from build123d import *

# Parameters (mm, degrees)
SKETCH2_R           = 2.15
BOSS_EXTRUDE1_DEPTH = 10.507214
CUT_EXTRUDE2_REACH  = 76.575
SKETCH4_R           = 2.15
CUT_EXTRUDE3_DEPTH  = 7
BOSS_EXTRUDE2_START = -7
SKETCH5_R           = 24.3
SKETCH5_R_2         = 23.3
BOSS_EXTRUDE2_DEPTH = 7
SKETCH6_R           = 23.3
CUT_EXTRUDE4_DEPTH  = 75.575465
CUT_EXTRUDE5_DEPTH  = 75.575465


with BuildPart() as part:
    # Sketch1 → Revolve1 (revolve)
    with BuildSketch(Plane(origin=(0, 0, 0), x_dir=(0, 0, -1), z_dir=(1, 0, 0)), mode=Mode.PRIVATE) as revolve1_sk:
        with BuildLine():
            Line((-37.5, -1.048229), (-37.5, -1.955443))
            Line((-37.5, -1.955443), (-25.283016, -1.955443))
            ThreePointArc((-25.283016, -1.955443), (-24.8, -2.421893), (-25.216498, -2.94859))
            ThreePointArc((-25.216498, -2.94859), (-25.276321, -2.982605), (-25.3, -3.04722))
            Line((-25.3, -3.04722), (-25.3, -4.555443))
            Line((-25.3, -4.555443), (-8, -4.555443))
            Line((-8, -4.555443), (-8, -11.555443))
            Line((-8, -11.555443), (-39.5, -11.555443))
            Line((-39.5, -11.555443), (-39.5, -1.048229))
            Line((-39.5, -1.048229), (-37.5, -1.048229))
        make_face()
    revolve(revolve1_sk.sketch.rotate(Axis((0, -1000, 0), (0, 1, 0)), 180), axis=Axis((0, -1000, 0), (0, 1, 0)))

    # Sketch2 → Boss-Extrude1 (add)
    # profile 1 of 4: a face of its own
    with BuildSketch(Plane.XZ.offset(11.555443)):
        with BuildLine():
            Line((-5, 47.5), (-5, 39.182266))
            Line((-5, 39.182266), (5, 39.182266))
            Line((5, 39.182266), (5, 47.5))
            ThreePointArc((5, 47.5), (0, 52.5), (-5, 47.5))
        make_face()
        with Locations(Location((0, 47.5, 0), (0, 0, 270))):
            Circle(SKETCH2_R, mode=Mode.SUBTRACT)
    # profile 2 of 4: a face of its own
    with BuildSketch(Plane.XZ.offset(11.555443)):
        with BuildLine():
            Line((47.5, -5), (39.182266, -5))
            Line((39.182266, -5), (39.182266, 5))
            Line((39.182266, 5), (47.5, 5))
            ThreePointArc((47.5, 5), (52.5, 0), (47.5, -5))
        make_face()
        with Locations(Location((47.5, 0, 0), (0, 0, 270))):
            Circle(SKETCH2_R, mode=Mode.SUBTRACT)
    # profile 3 of 4: a face of its own
    with BuildSketch(Plane.XZ.offset(11.555443)):
        with BuildLine():
            Line((-5, -47.5), (-5, -39.182266))
            Line((-5, -39.182266), (5, -39.182266))
            Line((5, -39.182266), (5, -47.5))
            ThreePointArc((5, -47.5), (0, -52.5), (-5, -47.5))
        make_face()
        with Locations(Location((0, -47.5, 0), (0, 0, 270))):
            Circle(SKETCH2_R, mode=Mode.SUBTRACT)
    # profile 4 of 4: a face of its own
    with BuildSketch(Plane.XZ.offset(11.555443)):
        with BuildLine():
            Line((-47.5, 5), (-39.182266, 5))
            Line((-39.182266, 5), (-39.182266, -5))
            Line((-39.182266, -5), (-47.5, -5))
            ThreePointArc((-47.5, -5), (-52.5, 0), (-47.5, 5))
        make_face()
        with Locations(Location((-47.5, 0, 0), (0, 0, 270))):
            Circle(SKETCH2_R, mode=Mode.SUBTRACT)
    extrude(amount=-BOSS_EXTRUDE1_DEPTH)

    # Sketch3 → Cut-Extrude2 (cut, up to next)
    with BuildSketch(Plane(origin=(0, -4.555443, 0), x_dir=(1, 0, 0), z_dir=(0, 1, 0)), mode=Mode.PRIVATE) as cut_extrude2_sk1:
        with BuildLine():
            Line((21.938323, -2), (12.369317, -2))
            ThreePointArc((12.369317, -2), (11.19262, -2.382785), (10.466345, -3.384615))
            ThreePointArc((10.466345, -3.384615), (7.778175, -7.778175), (3.384615, -10.466345))
            ThreePointArc((3.384615, -10.466345), (2.382785, -11.19262), (2, -12.369317))
            Line((2, -12.369317), (2, -21.938323))
            ThreePointArc((2, -21.938323), (2.718885, -23.474143), (4.358744, -23.905885))
            ThreePointArc((4.358744, -23.905885), (17.182695, -17.182695), (23.905885, -4.358744))
            ThreePointArc((23.905885, -4.358744), (23.474143, -2.718885), (21.938323, -2))
        make_face()
    cut_extrude2_tool1 = extrude(cut_extrude2_sk1.sketch, amount=-CUT_EXTRUDE2_REACH, mode=Mode.PRIVATE) & part.part
    # Sketch3 → Cut-Extrude2 (cut, up to next)
    with BuildSketch(Plane(origin=(0, -4.555443, 0), x_dir=(1, 0, 0), z_dir=(0, 1, 0)), mode=Mode.PRIVATE) as cut_extrude2_sk2:
        with BuildLine():
            Line((-2, -21.938323), (-2, -12.369317))
            ThreePointArc((-2, -12.369317), (-2.382785, -11.19262), (-3.384615, -10.466345))
            ThreePointArc((-3.384615, -10.466345), (-7.778175, -7.778175), (-10.466345, -3.384615))
            ThreePointArc((-10.466345, -3.384615), (-11.19262, -2.382785), (-12.369317, -2))
            Line((-12.369317, -2), (-21.938323, -2))
            ThreePointArc((-21.938323, -2), (-23.474143, -2.718885), (-23.905885, -4.358744))
            ThreePointArc((-23.905885, -4.358744), (-17.182695, -17.182695), (-4.358744, -23.905885))
            ThreePointArc((-4.358744, -23.905885), (-2.718885, -23.474143), (-2, -21.938323))
        make_face()
    cut_extrude2_tool2 = extrude(cut_extrude2_sk2.sketch, amount=-CUT_EXTRUDE2_REACH, mode=Mode.PRIVATE) & part.part
    # Sketch3 → Cut-Extrude2 (cut, up to next)
    with BuildSketch(Plane(origin=(0, -4.555443, 0), x_dir=(1, 0, 0), z_dir=(0, 1, 0)), mode=Mode.PRIVATE) as cut_extrude2_sk3:
        with BuildLine():
            Line((-21.938323, 2), (-12.369317, 2))
            ThreePointArc((-12.369317, 2), (-11.19262, 2.382785), (-10.466345, 3.384615))
            ThreePointArc((-10.466345, 3.384615), (-7.778175, 7.778175), (-3.384615, 10.466345))
            ThreePointArc((-3.384615, 10.466345), (-2.382785, 11.19262), (-2, 12.369317))
            Line((-2, 12.369317), (-2, 21.938323))
            ThreePointArc((-2, 21.938323), (-2.718885, 23.474143), (-4.358744, 23.905885))
            ThreePointArc((-4.358744, 23.905885), (-17.182695, 17.182695), (-23.905885, 4.358744))
            ThreePointArc((-23.905885, 4.358744), (-23.474143, 2.718885), (-21.938323, 2))
        make_face()
    cut_extrude2_tool3 = extrude(cut_extrude2_sk3.sketch, amount=-CUT_EXTRUDE2_REACH, mode=Mode.PRIVATE) & part.part
    # Sketch3 → Cut-Extrude2 (cut, up to next)
    with BuildSketch(Plane(origin=(0, -4.555443, 0), x_dir=(1, 0, 0), z_dir=(0, 1, 0)), mode=Mode.PRIVATE) as cut_extrude2_sk4:
        with BuildLine():
            Line((2, 21.938323), (2, 12.369317))
            ThreePointArc((2, 12.369317), (2.382785, 11.19262), (3.384615, 10.466345))
            ThreePointArc((3.384615, 10.466345), (7.778175, 7.778175), (10.466345, 3.384615))
            ThreePointArc((10.466345, 3.384615), (11.19262, 2.382785), (12.369317, 2))
            Line((12.369317, 2), (21.938323, 2))
            ThreePointArc((21.938323, 2), (23.474143, 2.718885), (23.905885, 4.358744))
            ThreePointArc((23.905885, 4.358744), (17.182695, 17.182695), (4.358744, 23.905885))
            ThreePointArc((4.358744, 23.905885), (2.718885, 23.474143), (2, 21.938323))
        make_face()
    cut_extrude2_tool4 = extrude(cut_extrude2_sk4.sketch, amount=-CUT_EXTRUDE2_REACH, mode=Mode.PRIVATE) & part.part
    add(cut_extrude2_tool1.solids().sort_by_distance((12.193258, -4.555443, 12.193258))[0], mode=Mode.SUBTRACT)
    add(cut_extrude2_tool2.solids().sort_by_distance((-12.193258, -4.555443, 12.193258))[0], mode=Mode.SUBTRACT)
    add(cut_extrude2_tool3.solids().sort_by_distance((-12.193258, -4.555443, -12.193258))[0], mode=Mode.SUBTRACT)
    add(cut_extrude2_tool4.solids().sort_by_distance((12.193258, -4.555443, -12.193258))[0], mode=Mode.SUBTRACT)

    # Sketch4 → Cut-Extrude3 (cut)
    with BuildSketch(Plane(origin=(0, -11.555443, 0), x_dir=(-1, 0, 0), z_dir=(0, -1, 0))):
        with Locations(Location((30, 0, 0), (0, 0, 90))):
            Circle(SKETCH4_R)
        with Locations(Location((0, -30, 0), (0, 0, 90))):
            Circle(SKETCH4_R)
        with Locations(Location((-30, 0, 0), (0, 0, 90))):
            Circle(SKETCH4_R)
        with Locations(Location((0, 30, 0), (0, 0, 90))):
            Circle(SKETCH4_R)
    extrude(amount=-CUT_EXTRUDE3_DEPTH, mode=Mode.SUBTRACT)

    # Sketch5 → Boss-Extrude2 (add)
    with BuildSketch(Plane.XZ.offset(11.555443).offset(BOSS_EXTRUDE2_START)):
        Circle(SKETCH5_R)
        Circle(SKETCH5_R_2, mode=Mode.SUBTRACT)
    extrude(amount=BOSS_EXTRUDE2_DEPTH)

    # Sketch6 → Cut-Extrude4 (cut, through all)
    with BuildSketch(Plane(origin=(0, -4.555443, 0), x_dir=(1, 0, 0), z_dir=(0, 1, 0))):
        with Locations(Location((0, 0, 0), (0, 0, 90))):
            Circle(SKETCH6_R)
    extrude(amount=-CUT_EXTRUDE4_DEPTH, mode=Mode.SUBTRACT)

    # Sketch7 → Cut-Extrude5 (cut, through all)
    with BuildSketch(Plane(origin=(0, -4.555443, 0), x_dir=(1, 0, 0), z_dir=(0, 1, 0))):
        with BuildLine():
            Line((11.65, 20.178392), (0, 0))
            Line((0, 0), (11.65, -20.178392))
            ThreePointArc((11.65, -20.178392), (20.178392, -11.65), (23.3, 0))
            ThreePointArc((23.3, 0), (20.178392, 11.65), (11.65, 20.178392))
        make_face()
        with BuildLine():
            Line((-11.65, -20.178392), (0, 0))
            Line((0, 0), (-11.65, 20.178392))
            ThreePointArc((-11.65, 20.178392), (-23.3, 0), (-11.65, -20.178392))
        make_face()
        with BuildLine():
            ThreePointArc((23.3, 0), (20.178392, -11.65), (11.65, -20.178392))
            Line((11.65, -20.178392), (12.65, -21.910443))
            ThreePointArc((12.65, -21.910443), (21.910443, -12.65), (25.3, 0))
            ThreePointArc((25.3, 0), (21.910443, 12.65), (12.65, 21.910443))
            Line((12.65, 21.910443), (11.65, 20.178392))
            ThreePointArc((11.65, 20.178392), (20.178392, 11.65), (23.3, 0))
        make_face()
        with BuildLine():
            Line((-12.65, -21.910443), (-11.65, -20.178392))
            ThreePointArc((-11.65, -20.178392), (-23.3, 0), (-11.65, 20.178392))
            Line((-11.65, 20.178392), (-12.65, 21.910443))
            ThreePointArc((-12.65, 21.910443), (-25.3, 0), (-12.65, -21.910443))
        make_face()
    extrude(amount=CUT_EXTRUDE5_DEPTH, mode=Mode.SUBTRACT)


solid = part.part
Could you check a few things on this model? Use its own coordinates, in mm. A direction names the side the tool comes from. Give positions to 0.01 mm unless a question says otherwise; leave off trailing zeros. Loops run counter-clockwise (first coordinate to the right, second up) from the corner with the lowest first, then second, coordinate; pieces in that order, holes last. Notation, with made-up numbers: (61.25, 32.25) -> (80.25, 32.25) arc R18 ccw to (80.25, 59.25) -> close; hole circle Ø2 at (37.5, 52). An arc over 180 degrees is marked (long way). Answer as CSV lines item,"result". Start each with the question number.
(1) If we section it at D-D on z = -30: Write out the boundary of the cut face in (x, y).
(2) I need wall thicknesses on probe 1 along X at (y, z) = (-1.6, 0); probe 2 along Y at (x, z) = (-29, 16.5); probe 3 along Z at (x, y) = (-32, -4.5). Which ranges of each line are inside material? Lowest first, please.
(3) Which directions (+Z, -Z, +X, -X, +Y, -Y) give clear straight access to the entire face, cutting with the end or side of a thin tool? Please do faces 1 (the cylindrical face through (33.27, -1.51, -17.3)), 2 (the cylindrical face through (-28.19, -8.1, -1.16)), 3 (the flat face through (-43, -6, -5)).
(4) If we section it at B-B on y = -6.25: Count the separate pieces of the cut face and the enclosed holes in it, then the cut area to 3 significant figures.
(5) If we section it at C-C on x = -30: Write out the boundary of the cut face in (y, z), then the cut area to 3 significant figures.
(6) We'd pull the mould along Z, two halves only. Please class faces 4 (the flat face through (5, -6, -43)), 5 (the flat face through (30, -4.555, 0)), 6 (the cylindrical face through (28.19, -6.23, -27.67)), 7 (the cylindrical face through (0.1, -6.4, 52.5)): released by +Z, released by -Z, zero draft, split by the parting line, or undercut.
(7) I'm going to push flat-ended pins straight in: pin 1 Ø15 at (x, z) = (17.5, -10.5) entering from +Y; pin 2 Ø1.5 at (x, y) = (-11.5, -8) entering from +Z; pin 3 Ø1.3 at (x, z) = (-29.5, -0.5) entering from -Y. Where does each tip first touch, or does it pass through?
(8) If we section it at A-A on z = 7.5: Write out the boundary of the cut face in (x, y).
Computed:
1,outline,"(-25.7, -11.56) -> (-2.15, -11.56) -> (-2.15, -4.56) -> (2.15, -4.56) -> (2.15, -11.56) -> (25.7, -11.56) -> (25.7, -1.05) -> (22.5, -1.05) -> (22.5, -1.96) -> (-22.5, -1.96) -> (-22.5, -1.05) -> (-25.7, -1.05) -> close"
2,probe 1,"x = -52.5 to -49.65, -45.35 to -37.5, 37.5 to 45.35, 49.65 to 52.5"
2,probe 2,"y = -11.56 to -1.96"
2,probe 3,"z = -23.16 to 23.16"
3,face 1,"+Y"
3,face 2,"-Y"
3,face 3,"-Z, -X, +Y, -Y"
4,separate pieces,"1"
4,enclosed holes,"9"
4,area,"3,560 mm2"
5,outline,"(-11.56, -25.7) -> (-1.05, -25.7) -> (-1.05, -22.5) -> (-1.96, -22.5) -> (-1.96, 22.5) -> (-1.05, 22.5) -> (-1.05, 25.7) -> (-11.56, 25.7) -> (-11.56, 2.15) -> (-4.56, 2.15) -> (-4.56, -2.15) -> (-11.56, -2.15) -> close"
5,area,"469 mm2"
6,face 4,"zero draft"
6,face 5,"undercut"
6,face 6,"released by -Z"
6,face 7,"released by +Z"
7,pin 1,"stops at y = -1.96"
7,pin 2,"stops at z = 38.01"
7,pin 3,"stops at y = -4.56"
8,outline,"(-38.78, -11.56) -> (-22.06, -11.56) -> (-22.06, -4.56) -> (-24.16, -4.56) -> (-24.16, -1.96) -> (-36.74, -1.96) -> (-36.74, -1.05) -> (-38.78, -1.05) -> close; (22.06, -11.56) -> (38.78, -11.56) -> (38.78, -1.05) -> (36.74, -1.05) -> (36.74, -1.96) -> (24.16, -1.96) -> (24.16, -4.56) -> (22.06, -4.56) -> close"
